from build123d import *

# Parameters (mm, degrees)
CROQUIS1_W              = 98
CROQUIS1_H              = 45
SALIENTE_EXTRUIR1_DEPTH = 34
REDONDEO1_R             = 5
CROQUIS2_R              = 4.125
CROQUIS2_R_2            = 2.5
CORTAR_EXTRUIR1_DEPTH   = 8
CORTAR_EXTRUIR2_DEPTH   = 18
CROQUIS4_W              = 39
CROQUIS4_H              = 3
SALIENTE_EXTRUIR2_DEPTH = 12
CROQUIS5_R              = 3.54232781
CORTAR_EXTRUIR3_DEPTH   = 21


with BuildPart() as part:
    # Croquis1 → Saliente-Extruir1 (new body)
    with BuildSketch(Plane(origin=(0, 0, 0), x_dir=(0, 1, 0), z_dir=(0, 0, 1))):
        Rectangle(CROQUIS1_W, CROQUIS1_H)
    extrude(amount=SALIENTE_EXTRUIR1_DEPTH)

    # Redondeo1
    redondeo1_edges = [part.edges().sort_by_distance(p)[0] for p in [
        (22.5, 49, 17),
        (22.5, -49, 17),
        (-22.5, -49, 17),
        (-22.5, 49, 17),
    ]]
    fillet(redondeo1_edges, radius=REDONDEO1_R)

    # Croquis2 → Cortar-Extruir1 (cut)
    with BuildSketch(Plane.XY.offset(34)):
        with Locations((0, 43)):
            Circle(CROQUIS2_R)
        with Locations((0, -43)):
            Circle(CROQUIS2_R)
        with Locations((-11.225, 43)):
            Circle(CROQUIS2_R_2)
        with Locations((11.225, -43)):
            Circle(CROQUIS2_R_2)
    extrude(amount=-CORTAR_EXTRUIR1_DEPTH, mode=Mode.SUBTRACT)

    # Croquis3 → Cortar-Extruir2 (cut)
    with BuildSketch(Plane.XY.offset(34)):
        with BuildLine():
            Line((-19.5, -35), (-19.5, 35))
            ThreePointArc((-19.5, 35), (-18.914213562, 36.414213562), (-17.5, 37))
            Line((-17.5, 37), (17.5, 37))
            ThreePointArc((17.5, 37), (18.914213562, 36.414213562), (19.5, 35))
            Line((19.5, 35), (19.5, 31.792704716))
            Line((19.5, 31.792704716), (22.5, 31.792704716))
            Line((22.5, 31.792704716), (22.5, 4.207295284))
            Line((22.5, 4.207295284), (19.5, 4.207295284))
            Line((19.5, 4.207295284), (19.5, -4.207295284))
            Line((19.5, -4.207295284), (22.5, -4.207295284))
            Line((22.5, -4.207295284), (22.5, -31.792704716))
            Line((22.5, -31.792704716), (19.5, -31.792704716))
            Line((19.5, -31.792704716), (19.5, -35))
            ThreePointArc((19.5, -35), (18.914213562, -36.414213562), (17.5, -37))
            Line((17.5, -37), (-17.5, -37))
            ThreePointArc((-17.5, -37), (-18.914213562, -36.414213562), (-19.5, -35))
        make_face()
    extrude(amount=-CORTAR_EXTRUIR2_DEPTH, mode=Mode.SUBTRACT)

    # Croquis4 → Saliente-Extruir2 (add)
    with BuildSketch(Plane.XY.offset(16)):
        Rectangle(CROQUIS4_W, CROQUIS4_H)
    extrude(amount=SALIENTE_EXTRUIR2_DEPTH)

    # Croquis5 → Cortar-Extruir3 (cut)
    with BuildSketch(Plane(origin=(-22.5, 0, 0), x_dir=(0, -1, 0), z_dir=(-1, 0, 0))):
        with Locations(Location((-7.749623094, 8, 0), (0, 0, 90))):
            Circle(CROQUIS5_R)
        with Locations(Location((-18, 8, 0), (0, 0, 90))):
            Circle(CROQUIS5_R)
        with Locations(Location((-28.250376906, 8, 0), (0, 0, 90))):
            Circle(CROQUIS5_R)
        with Locations(Location((28.250376906, 8, 0), (0, 0, 270))):
            Circle(CROQUIS5_R)
        with Locations(Location((18, 8, 0), (0, 0, 270))):
            Circle(CROQUIS5_R)
        with Locations(Location((7.749623094, 8, 0), (0, 0, 270))):
            Circle(CROQUIS5_R)
    extrude(amount=-CORTAR_EXTRUIR3_DEPTH, mode=Mode.SUBTRACT)


solid = part.part
Verification items for the finished model (mm, model axes). A direction names the side the tool comes from. Round coordinates to 2 decimals unless told otherwise and drop trailing zeros. Write each loop counter-clockwise with the first axis right and the second up, starting at its lowest first coordinate (ties: lowest second). Pieces come first, ordered by that corner, then holes.
(1) Material ranges on line 1 (Y direction, x = 17.5, z = 20); line 2 (X direction, y = -34, z = 27.5); line 3 (Z direction, x = 10.5, y = -44.5), recorded low to high.
Returned:
line 1: y = -49 to -37, -1.5 to 1.5, 37 to 49
line 2: x = -22.5 to -19.5, 19.5 to 22.5
line 3: z = 0 to 26
(2) Section check C-C (x = 0). Enter the section's corners in (y, z) (3 decimals).
Returned:
outline: (-49, 0) - (49, 0) - (49, 34) - (47.125, 34) - (47.125, 26) - (38.875, 26) - (38.875, 34) - (37, 34) - (37, 16) - (1.5, 16) - (1.5, 28) - (-1.5, 28) - (-1.5, 16) - (-37, 16) - (-37, 34) - (-38.875, 34) - (-38.875, 26) - (-47.125, 26) - (-47.125, 34) - (-49, 34) - close
(3) Section check D-D (x = -12.5). Enter the section's corners in (y, z).
Returned:
outline: (-49, 0) - (49, 0) - (49, 34) - (45.15, 34) - (45.15, 26) - (40.85, 26) - (40.85, 34) - (37, 34) - (37, 16) - (1.5, 16) - (1.5, 28) - (-1.5, 28) - (-1.5, 16) - (-37, 16) - (-37, 34) - (-49, 34) - close; hole circle Ø7.08 at (-28.25, 8); hole circle Ø7.08 at (-18, 8); hole circle Ø7.08 at (-7.75, 8); hole circle Ø7.08 at (7.75, 8); hole circle Ø7.08 at (18, 8); hole circle Ø7.08 at (28.25, 8)
(4) Depth check by flat-ended pin: pin 1 Ø2.5 at (x, z) = (21.5, 27.5) entering from +Y; pin 2 Ø5.5 at (y, z) = (17.5, 26.5) entering from +X; pin 3 Ø1.5 at (x, y) = (8.5, 0) entering from +Z. Enter the tip coordinate at first touch or a pass-through.
Returned:
pin 1: stops at y = 48.18
pin 2: stops at x = -19.5
pin 3: stops at z = 28
(5) Access from +Z, -Z, +X, -X, +Y, -Y to the whole of each face (thin tool, end or side, straight path). Record for faces 1 (the cylindrical face through (-12.15, 20.99, 9.9)), 2 (the flat face through (0, 49, 17)), 3 (the flat face through (-11, 43, 26)).
Returned:
face 1: -X
face 2: +Z, -Z, +X, -X, +Y
face 3: +Z
(6) Section check B-B (y = -43). Enter the section's corners in (x, z) (3 decimals).
Returned:
outline: (-22.5, 0) - (22.5, 0) - (22.5, 34) - (13.725, 34) - (13.725, 26) - (8.725, 26) - (8.725, 34) - (4.125, 34) - (4.125, 26) - (-4.125, 26) - (-4.125, 34) - (-22.5, 34) - close
(7) Mould release check, pull along X, two halves, no side actions. Record for faces 4 (the cylindrical face through (-21, 47.57, 17.24)), 5 (the cylindrical face through (-18.9, -36.43, 25.13)), 6 (the cylindrical face through (10.68, -45.44, 30.06)), 7 (the flat face through (21, 4.207, 25)): pulls with the +X half, pulls with the -X half, needs draft (parallel to the pull), parting line crosses it, or undercut.
Returned:
face 4: pulls with the -X half
face 5: undercut
face 6: undercut
face 7: needs draft
